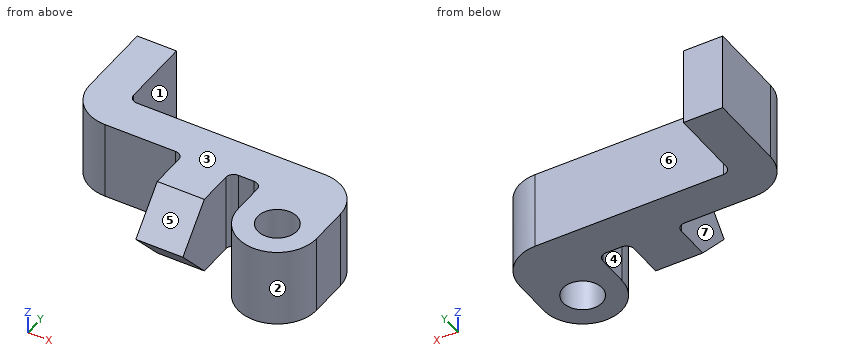
```python
from build123d import *

# Parameters (mm, degrees)
F0_R     = 2.5
F1_DEPTH = 10
F2_R     = 5
F3_R     = 1
F5_DEPTH = 6


with BuildPart() as f1:
    # F0 (on Top) → F1 (new body)
    with BuildSketch(Plane.XY):
        with BuildLine():
            Line((0, 25), (0, 10))
            Line((0, 10), (15, 10))
            Line((15, 10), (15, 0))
            Line((15, 0), (21, 0))
            Line((21, 0), (21, 10))
            Line((21, 10), (25, 10))
            Line((25, 10), (25, 5))
            ThreePointArc((25, 5), (30, 0), (35, 5))
            Line((35, 5), (35, 15))
            Line((35, 15), (5, 15))
            Line((5, 15), (5, 25))
            Line((5, 25), (0, 25))
        make_face()
        with Locations((30, 5)):
            Circle(F0_R, mode=Mode.SUBTRACT)
    extrude(amount=F1_DEPTH)

    # F2
    f2_edges = [f1.edges().sort_by_distance(p)[0] for p in [
        (0, 10, 5),
        (35, 15, 5),
    ]]
    fillet(f2_edges, radius=F2_R)

    # F3
    f3_edges = [f1.edges().sort_by_distance(p)[0] for p in [
        (15, 10, 5),
        (5, 15, 5),
        (25, 10, 5),
        (21, 10, 5),
    ]]
    fillet(f3_edges, radius=F3_R)

    # F4 (on face) → F5 (cut)
    with BuildSketch(Plane(origin=(15, 0, 0), x_dir=(0, -1, 0), z_dir=(-1, 0, 0))):
        Polygon((-4.5, 10), (0, 5), (0, 10), align=None)
        Polygon((0, 5), (-4.5, 0), (0, 0), align=None)
    extrude(amount=-F5_DEPTH, mode=Mode.SUBTRACT)


solid = f1.part
```
Can you work these out from the model? Positions are in its coordinate system, mm. Face numbers are marked on the shaded views. A direction names the side the tool comes from. Round coordinates to 2 decimals unless told otherwise and drop trailing zeros. Order: outer loops, then holes, each group sorted by start corner. A loop starts at its lowest first (then second) coordinate and runs counter-clockwise, first axis right, second up. Notation, with made-up numbers: (68, 48.25) -> (123, 48.25) arc R26 cw to (123, 66.25) -> close; hole circle Ø4 at (-15.5, -13.5). An arc over 180 degrees is marked (long way). Return JSON: item names as keys, results as strings. Group by question number.
1. Will these pins go through, and if not, where does the flat tip stop? pin 1 (4 mm diameter, centred on y = 13, z = 5.5, fed in from +X); pin 2 (2 mm diameter, centred on y = 16.5, z = 8, fed in from +X); pin 3 (3 mm diameter, centred on y = 7.5, z = 4.5, fed in from -X).
2. If we section it at A-A, the plane z = 3.5: Write out the boundary of the cut face in (x, y).
3. If we section it at C-C, the plane y = 21.5: Write out the boundary of the cut face in (x, z).
4. We'd pull the mould along X, two halves only. Please class the marked faces 1, 2 and 3: released by +X, released by -X, zero draft, split by the parting line, or undercut.
5. I need wall thicknesses on line 1 (X direction, y = 9, z = 1.75); line 2 (Y direction, x = 30, z = 5.25); line 3 (X direction, y = 4.25, z = 2). Which ranges of each line are inside material? Lowest first, please. Write a range as [from, to].
6. If we section it at D-D, the plane z = 5.5: Write out the boundary of the cut face in (x, y), then the cut area to 3 significant figures.
7. Which directions (+Z, -Z, +X, -X, +Y, -Y) give clear straight access to the entire face, cutting with the end or side of a thin tool? Please do the marked faces 4, 5, 6 and 7.
8. If we section it at B-B, the plane x = 19: Write out the boundary of the cut face in (y, z).
Output values:
{
 "1": {"pin 1": "x = 34.9", "pin 2": "x = 5.13", "pin 3": "x = 15"},
 "2": {"outline": "(0, 15) arc R5 ccw to (5, 10) -> (14, 10) arc R1 cw to (15, 9) -> (15, 1.35) -> (21, 1.35) -> (21, 9) arc R1 cw to (22, 10) -> (24, 10) arc R1 cw to (25, 9) -> (25, 5) arc R5 ccw to (35, 5) -> (35, 10) arc R5 ccw to (30, 15) -> (6, 15) arc R1 cw to (5, 16) -> (5, 25) -> (0, 25) -> close; hole circle Ø5 at (30, 5)"},
 "3": {"outline": "(0, 0) -> (5, 0) -> (5, 10) -> (0, 10) -> close"},
 "4": {"face 1": "released by +X", "face 2": "undercut", "face 3": "zero draft"},
 "5": {"line 1": "[15, 21], [25, 35]", "line 2": "[0, 2.5], [7.5, 15]", "line 3": "[15, 21], [25.06, 27.62], [32.38, 34.94]"},
 "6": {"outline": "(0, 15) arc R5 ccw to (5, 10) -> (14, 10) arc R1 cw to (15, 9) -> (15, 0.45) -> (21, 0.45) -> (21, 9) arc R1 cw to (22, 10) -> (24, 10) arc R1 cw to (25, 9) -> (25, 5) arc R5 ccw to (35, 5) -> (35, 10) arc R5 ccw to (30, 15) -> (6, 15) arc R1 cw to (5, 16) -> (5, 25) -> (0, 25) -> close; hole circle Ø5 at (30, 5)", "area": "342 mm²"},
 "7": {"face 4": "+Z, -Z, -Y", "face 5": "+Z, -X, -Y", "face 6": "+Z, -Z, +X, +Y", "face 7": "+Z, -Z, -X, -Y"},
 "8": {"outline": "(0, 5) -> (4.5, 0) -> (15, 0) -> (15, 10) -> (4.5, 10) -> close"}
}
